from build123d import *

# Parameters (mm, degrees)
SKETCH1_W           = 28
SKETCH1_H           = 15
BOSS_EXTRUDE1_DEPTH = 5
SKETCH2_W           = 0.4
SKETCH2_H           = 0.4
SKETCH2_W_2         = 0.6
SKETCH2_H_2         = 1
BOSS_EXTRUDE2_DEPTH = 4.3


with BuildPart() as part:
    # Sketch1 → Boss-Extrude1 (new body)
    with BuildSketch(Plane(origin=(0, 0, 0), x_dir=(0, 0, -1), z_dir=(1, 0, 0))):
        with Locations((14, 7.5)):
            Rectangle(SKETCH1_W, SKETCH1_H)
    extrude(amount=BOSS_EXTRUDE1_DEPTH)

    # Sketch2 → Boss-Extrude2 (add)
    with BuildSketch(Plane.XZ):
        with Locations((1.2, -1.2)):
            Rectangle(SKETCH2_W, SKETCH2_H)
        with Locations((1.2, -4.8)):
            Rectangle(SKETCH2_W, SKETCH2_H)
        with Locations((1.3, -26.1)):
            Rectangle(SKETCH2_W_2, SKETCH2_H_2)
        with Locations((1.3, -21.1)):
            Rectangle(SKETCH2_W_2, SKETCH2_H_2)
        with Locations((1.3, -16.1)):
            Rectangle(SKETCH2_W_2, SKETCH2_H_2)
    extrude(amount=BOSS_EXTRUDE2_DEPTH)


solid = part.part
CAD build for the part. Positions are in the model's coordinates, mm. A direction names the side the tool comes from. Give positions to 0.01 mm unless a question says otherwise; leave off trailing zeros. Order: outer loops, then holes, each group sorted by start corner. A loop starts at its lowest first (then second) coordinate and runs counter-clockwise, first axis right, second up. Notation, with made-up numbers: (0, 28.25) - (43, 28.25) arc R28 cw to (43, 60.25) - close; hole circle Ø2 at (-27, 73.5). An arc over 180 degrees is marked (long way). Answer in a Markdown table with one row per item.
1. Probe probe 1 along Y at (x, z) = (1.4, -1.5); probe 2 along X at (y, z) = (-0.5, -21.5). List the from-to ranges inside material, lowest first. Write a range as [from, to].
Data:
| item | result |
|---|---|
| probe 1 | y = [0, 15] |
| probe 2 | x = [1, 1.6] |
2. Saw through at B-B, the plane z = -5.5. Give the cut face in (x, y).
Data:
| item | result |
|---|---|
| outline | (0, 0) - (5, 0) - (5, 15) - (0, 15) - close |
3. Flat gauge pins, fed straight in: pin 1 (0.5 mm diameter, centred on x = 1.5, y = -2.5, fed in from +Z); pin 2 (0.5 mm diameter, centred on x = 1.5, y = -1, fed in from -Z); pin 3 (0.8 mm diameter, centred on y = -3, z = -21, fed in from +X). Where does each tip first touch, or does it go through?
Data:
| item | result |
|---|---|
| pin 1 | stops at z = -1 |
| pin 2 | stops at z = -26.6 |
| pin 3 | stops at x = 1.6 |
4. Tool access for faces 1 (the flat face through (2, 7, 0)), 2 (the flat face through (1, -2, -26)), 3 (the flat face through (1.6, -2, -21)): list every direction of +Z, -Z, +X, -X, +Y, -Y with a clear straight run to the whole face (end or side of a thin tool).
Data:
| item | result |
|---|---|
| face 1 | +Z, +X, -X, +Y, -Y |
| face 2 | +Z, -Z, -X, -Y |
| face 3 | +Z, -Z, +X, -Y |
5. Saw through at A-A, the plane x = 4.65. Give the cut face in (y, z), plus the area to 3 significant figures.
Data:
| item | result |
|---|---|
| outline | (0, -28) - (15, -28) - (15, 0) - (0, 0) - close |
| area | 420 mm² |
